```python
from build123d import *

# Parameters (mm, degrees)
SKETCH_1_W          = 115.019292035
SKETCH_1_H          = 22.927433628
EXTRUDE_1_DEPTH     = 14.986
SKETCH_2_R          = 2.628127437
EXTRUDE_2_DEPTH     = 7.366
EXTRUDE_3_DEPTH     = 2.54
EXTRUDE_4_DEPTH     = 2.794
SKETCH_6_R          = 1.611317842
EXTRUDE_5_DEPTH     = 0.508
EXTRUDE_6_DEPTH     = 4.064
SKETCH_8_W          = 20.74444914
SKETCH_8_H          = 3.147990337
SKETCH_8_H_2        = 3.147990336
EXTRUDE_7_DEPTH     = 10.922
SKETCH_9_W          = 20.74444914
SKETCH_9_H          = 1.904400454
EXTRUDE_8_DEPTH     = 10.922
SKETCH_10_R         = 2.28563118
EXTRUDE_9_DEPTH     = 0.762
SKETCH_11_R         = 1.571986642
EXTRUDE_10_DEPTH    = 3.302
SKETCH_12_W         = 17.575344956
SKETCH_12_H         = 16.755162191
EXTRUDE_11_DEPTH    = 13.462
SKETCH_13_R         = 1.331265642
SKETCH_13_R_2       = 1.077265642
CUT_EXTRUDE_1_DEPTH = 0.762
SKETCH_14_W         = 16.834327137
SKETCH_14_H         = 20.427018904
CUT_EXTRUDE_2_DEPTH = 28.194


with BuildPart() as part:
    # 草图1 → 凸台-拉伸1 (new body)
    with BuildSketch(Plane.XY):
        with Locations((14.25011379, -11.463716814)):
            Rectangle(SKETCH_1_W, SKETCH_1_H)
    extrude(amount=EXTRUDE_1_DEPTH)

    # 草图2 → 凸台-拉伸2 (add)
    with BuildSketch(Plane.XY.offset(14.986)):
        with Locations((58.785943209, -11.743523072)):
            Circle(SKETCH_2_R)
    extrude(amount=EXTRUDE_2_DEPTH)

    # 草图3 → 凸台-拉伸3 (add)
    with BuildSketch(Plane.XY.offset(21.844)):
        with BuildLine():
            Line((53.76517402, -10.973439102), (53.706459714, -11.743523072))
            ThreePointArc((53.706459714, -11.743523072), (58.785943209, -16.823006567), (63.865426703, -11.743523072))
            Line((63.865426703, -11.743523072), (63.806712398, -10.973439102))
            Line((63.806712398, -10.973439102), (61.171013627, 23.595808677))
            ThreePointArc((61.171013627, 23.595808677), (58.785943209, 25.980879095), (56.400872791, 23.595808677))
            Line((56.400872791, 23.595808677), (53.76517402, -10.973439102))
        make_face()
    extrude(amount=-EXTRUDE_3_DEPTH)

    # 草图5 → 凸台-拉伸4 (add)
    with BuildSketch(Plane(origin=(0, 0, 19.304), x_dir=(-1, 0, 0), z_dir=(0, 0, -1))):
        with BuildLine():
            Line((-57.536519865, 25.108887591), (-13.949230135, -10.883271683))
            ThreePointArc((-13.949230135, -10.883271683), (-13.53146296, -16.06321478), (-18.721435344, -16.328783135))
            Line((-18.721435344, -16.328783135), (-60.121986544, 22.158639689))
            ThreePointArc((-60.121986544, 22.158639689), (-60.261702819, 24.88909908), (-57.536519865, 25.108887591))
        make_face()
    extrude(amount=EXTRUDE_4_DEPTH)

    # 草图6 → 凸台-拉伸5 (add)
    with BuildSketch(Plane.XY.offset(21.844)):
        with Locations((58.785943209, 23.595808677)):
            Circle(SKETCH_6_R)
    extrude(amount=EXTRUDE_5_DEPTH)

    # 草图7 → 凸台-拉伸6 (add)
    with BuildSketch(Plane.XY.offset(19.304)):
        with BuildLine():
            Line((16.255391973, -10.80751129), (-72.73334393, -10.80751129))
            Line((-72.73334393, -10.80751129), (-72.73334393, -16.544656626))
            Line((-72.73334393, -16.544656626), (16.255391973, -16.544656626))
            ThreePointArc((16.255391973, -16.544656626), (19.123964641, -13.676083958), (16.255391973, -10.80751129))
        make_face()
    extrude(amount=EXTRUDE_6_DEPTH)

    # 草图8 → 凸台-拉伸7 (add)
    with BuildSketch(Plane.XY.offset(14.986)):
        with Locations((-27.006170601, -20.578235082)):
            Rectangle(SKETCH_8_W, SKETCH_8_H)
        with Locations((-27.006170601, -6.773932835)):
            Rectangle(SKETCH_8_W, SKETCH_8_H_2)
    extrude(amount=EXTRUDE_7_DEPTH)

    # 草图9 → 凸台-拉伸8 (add)
    with BuildSketch(Plane.XZ.offset(8.347928003)):
        with Locations((-27.006170601, 24.955799773)):
            Rectangle(SKETCH_9_W, SKETCH_9_H)
    extrude(amount=EXTRUDE_8_DEPTH)

    # 草图10 → 凸台-拉伸9 (add)
    with BuildSketch(Plane.XY.offset(23.368)):
        with Locations(Location((16.302879151, -13.669496202, 0), (0, 0, 180))):
            Circle(SKETCH_10_R)
    extrude(amount=EXTRUDE_9_DEPTH)

    # 草图11 → 凸台-拉伸10 (add)
    with BuildSketch(Plane(origin=(0, 0, 0), x_dir=(-1, 0, 0), z_dir=(0, 0, -1))):
        with Locations(Location((-59.445134238, -13.353735996, 0), (0, 0, 180))):
            Circle(SKETCH_11_R)
    extrude(amount=EXTRUDE_10_DEPTH)

    # 草图12 → 凸台-拉伸11 (add)
    with BuildSketch(Plane(origin=(0, 0, -3.302), x_dir=(-1, 0, 0), z_dir=(0, 0, -1))):
        with Locations((-59.093627339, -14.115334278)):
            Rectangle(SKETCH_12_W, SKETCH_12_H)
    extrude(amount=EXTRUDE_11_DEPTH)

    # 草图13 → 切除-拉伸1 (cut)
    with BuildSketch(Plane(origin=(0, 0, 16.51), x_dir=(-1, 0, 0), z_dir=(0, 0, -1))):
        with Locations((-58.850171018, 23.520615078)):
            Circle(SKETCH_13_R)
        with Locations((-58.850171018, 23.520615078)):
            Circle(SKETCH_13_R_2, mode=Mode.SUBTRACT)
    extrude(amount=-CUT_EXTRUDE_1_DEPTH, mode=Mode.SUBTRACT)

    # 草图14 → 切除-拉伸2 (cut)
    with BuildSketch(Plane(origin=(67.881299817, 0, 0), x_dir=(0, 0, -1), z_dir=(1, 0, 0))):
        with Locations((11.672099204, -13.921851865)):
            Rectangle(SKETCH_14_W, SKETCH_14_H)
    extrude(amount=-CUT_EXTRUDE_2_DEPTH, mode=Mode.SUBTRACT)


solid = part.part
```
Here's how the part is built. I have some questions about the finished solid (model axes, mm). A direction names the side the tool comes from. Give positions to 0.01 mm unless a question says otherwise; leave off trailing zeros. Order: outer loops, then holes, each group sorted by start corner. A loop starts at its lowest first (then second) coordinate and runs counter-clockwise, first axis right, second up. Notation, with made-up numbers: M 56,64.25 L 88,64.25 A17 cw 88,86.25 Z; hole C -19.75,17.5 d5. An arc over 180 degrees is marked long. Use a Markdown table: item, result. Add a question column.
1. Suppose I cut it at D-D (y = 1.5). List the corners of the cut face in (x, z) for me.
2. Suppose I cut it at C-C (y = -7). List the corners of the cut face in (x, z) for me, and give its area (3 significant figures).
3. Suppose I cut it at A-A (x = -34.5). List the corners of the cut face in (y, z) for me.
4. Suppose I cut it at B-B (x = 43.5). List the corners of the cut face in (y, z) for me, and give its area (3 significant figures).
5. If we mould it in two halves opening along X, with no side actions, what happens to faces 5 (the cylindrical face through (61.214, -12.75, 17.115)), 6 (the flat face through (-29, -16.545, 21)), 7 (the cylindrical face through (59.529, 22.166, 22.094))? For each: +X half, -X half, draft (parallel to the pull), parting line (faces both ways), or undercut.
6. I need wall thicknesses on probe 1 along Y at (x, z) = (15.5, 20.5); probe 2 along Z at (x, y) = (44, -4.5); probe 3 along X at (y, z) = (-14.5, 4.25). Which ranges of each line are inside material? Lowest first, please. Write a range as from..to.
7. For pin 1 Ø4.5 at (x, y) = (-4.5, -13.5) entering from +Z; pin 2 Ø8.5 at (y, z) = (-12.5, 21) entering from +X; pin 3 Ø5 at (x, y) = (55, -10.5) entering from +Z, each with a flat end and sliding along its axis, tell me the tip position at first contact or that it passes through.
8. On a 3-axis mill with a long thin cutter (end or side, diameter ignored), from which of +Z, -Z, +X, -X, +Y, -Y can I reach the whole of each face in a straight line? I mean faces 1 (the flat face through (16, -14, 24.13)), 2 (the flat face through (-27, -22.152, 20)), 3 (the cylindrical face through (19.123, -13.739, 21.308)), 4 (the flat face through (-27, -8.348, 19)). Say none if no direction works.
Results list:
| question | item | result |
|---|---|---|
| 1 | outline | M 28.95,16.51 L 37.9,16.51 L 37.9,19.3 L 28.95,19.3 Z; M 54.72,19.3 L 62.86,19.3 L 62.86,21.84 L 54.72,21.84 Z |
| 2 | outline | M -43.26,0 L 71.76,0 L 71.76,14.99 L -16.63,14.99 L -16.63,25.91 L -37.38,25.91 L -37.38,14.99 L -43.26,14.99 Z; M 18.65,16.51 L 28.76,16.51 L 28.76,19.3 L 18.65,19.3 Z; M 54.07,19.3 L 63.5,19.3 L 63.5,21.84 L 54.07,21.84 Z |
| 2 | area | 2,000 mm² |
| 3 | outline | M -22.93,0 L 0,0 L 0,14.99 L -5.2,14.99 L -5.2,25.91 L -22.15,25.91 L -22.15,14.99 L -22.93,14.99 Z; M -16.54,19.3 L -10.81,19.3 L -10.81,23.37 L -16.54,23.37 Z; hole M -19,14.99 L -8.35,14.99 L -8.35,24 L -19,24 Z |
| 4 | outline | M -22.93,0 L 0,0 L 0,14.99 L -22.93,14.99 Z; M 6.71,16.51 L 13.52,16.51 L 13.52,19.3 L 6.71,19.3 Z |
| 4 | area | 363 mm² |
| 5 | face 5 | undercut |
| 5 | face 6 | draft |
| 5 | face 7 | parting line |
| 6 | probe 1 | y = -16.54..-10.81 |
| 6 | probe 2 | z = 0..14.99 |
| 6 | probe 3 | x = -43.26..71.76 |
| 7 | pin 1 | stops at z = 23.37 |
| 7 | pin 2 | stops at x = 63.87 |
| 7 | pin 3 | stops at z = 22.35 |
| 8 | face 1 | +Z, +X, +Y, -Y |
| 8 | face 2 | +Z, +X, -X, -Y |
| 8 | face 3 | +Z |
| 8 | face 4 | -X |
